```python
from build123d import *

# Parameters (mm, degrees)
SKETCH_1_W         = 90
SKETCH_1_H         = 110
EXTRUDE_1_DEPTH    = 5
CHAMFER_1_SIZE     = 10
HOLE_WIZARD_M3_1_D = 2.5


with BuildPart() as part:
    # 草图1 → 凸台-拉伸1 (new body)
    with BuildSketch(Plane(origin=(0, 0, 0), x_dir=(1, 0, 0), z_dir=(0, 1, 0))):
        with Locations((45, 55)):
            Rectangle(SKETCH_1_W, SKETCH_1_H)
    extrude(amount=EXTRUDE_1_DEPTH)

    # 倒角1
    chamfer_1_edges = [part.edges().sort_by_distance(p)[0] for p in [
        (0, 2.5, 0),
        (0, 2.5, -110),
        (90, 2.5, -110),
        (90, 2.5, 0),
    ]]
    chamfer(chamfer_1_edges, length=CHAMFER_1_SIZE)

    # M3 螺纹孔1 (through all)
    with Locations(Plane(origin=(0, 0, 0), x_dir=(-1, 0, 0), z_dir=(0, -1, 0))):
        with Locations((-19, 78.5), (-19, 31.5), (-32, 31.5), (-32, 78.5)):
            Hole(HOLE_WIZARD_M3_1_D / 2)


solid = part.part
```
Part model, mm, in its own coordinate system. Round coordinates to 2 decimals unless told otherwise and drop trailing zeros. Write each loop counter-clockwise with the first axis right and the second up, starting at its lowest first coordinate (ties: lowest second). Pieces come first, ordered by that corner, then holes.
Item 1: Cut at A-A, the plane z = -31.5. Give the cut face in (x, y), plus the area to 3 significant figures.
Results:
outline: (0, 0) - (17.75, 0) - (17.75, 5) - (0, 5) - close; (20.25, 0) - (30.75, 0) - (30.75, 5) - (20.25, 5) - close; (33.25, 0) - (90, 0) - (90, 5) - (33.25, 5) - close
area: 425 mm2
Item 2: Two-plate mould, pull along X, no slides. Class faces 1 (the flat face through (45, 2, 0)), 2 (the cylindrical face through (18.84, 2.53, -79.74)), 3 (the flat face through (0, 2, -54)): +X half, -X half, draft (parallel to the pull), parting line (faces both ways), or undercut.
Results:
face 1: draft
face 2: undercut
face 3: -X half
Item 3: Cut at C-C, the plane y = 2.35. Give the cut face in (x, z).
Results:
outline: (0, -100) - (10, -110) - (80, -110) - (90, -100) - (90, -10) - (80, 0) - (10, 0) - (0, -10) - close; hole circle Ø2.5 at (19, -78.5); hole circle Ø2.5 at (19, -31.5); hole circle Ø2.5 at (32, -78.5); hole circle Ø2.5 at (32, -31.5)
Item 4: Cut at D-D, the plane z = -102.5. Give the cut face in (x, y).
Results:
outline: (2.5, 0) - (87.5, 0) - (87.5, 5) - (2.5, 5) - close
Item 5: Probe L1, parallel to Z at x = 19, y = 3.8; L2, parallel to X at y = 2.75, z = -78.5; L3, parallel to Z at x = 31, y = 0.55. List the from-to ranges inside material, lowest first.
Results:
L1: z = -110 to -79.75, -77.25 to -32.75, -30.25 to 0
L2: x = 0 to 17.75, 20.25 to 30.75, 33.25 to 90
L3: z = -110 to -79.25, -77.75 to -32.25, -30.75 to 0
Item 6: Drop a flat-ended pin along its axis: pin 1 Ø4 at (x, z) = (32, -78.5) entering from -Y. Give the stop position or say it passes through.
Results:
pin 1: stops at y = 0
Item 7: Cut at B-B, the plane x = 19. Give the cut face in (y, z), plus the area to 3 significant figures.
Results:
outline: (0, -110) - (5, -110) - (5, -79.75) - (0, -79.75) - close; (0, -77.25) - (5, -77.25) - (5, -32.75) - (0, -32.75) - close; (0, -30.25) - (5, -30.25) - (5, 0) - (0, 0) - close
area: 525 mm2
